Could you check a few things on this model? Use its own coordinates, in mm. Face numbers are marked on the shaded views. A direction names the side the tool comes from. Give positions to 0.01 mm unless a question says otherwise; leave off trailing zeros. Loops run counter-clockwise (first coordinate to the right, second up) from the corner with the lowest first, then second, coordinate; pieces in that order, holes last. Notation, with made-up numbers: (39, -7) - (78, -7) arc R31 cw to (78, 31) - close; hole circle Ø2 at (51, 52.5). An arc over 180 degrees is marked (long way). Write each question's results on one line, items separated by ' | '. Start each with the question number.
1) I'm going to push flat-ended pins straight in: pin 1 (1.1 mm diameter, centred on x = -1, z = 4.5, fed in from +Y); pin 2 (3 mm diameter, centred on x = 3, z = 1.5, fed in from +Y); pin 3 (0.8 mm diameter, centred on y = -1.5, z = 4.5, fed in from -X). Where does each tip first touch, or does it pass through?
2) If we mould it in two halves opening along Y, with no side actions, what happens to the marked faces 4, 5 and 6? For each: +Y half, -Y half, draft (parallel to the pull), parting line (faces both ways), or undercut.
3) I want a section at A-A, the plane z = 1.05. Write out the boundary of the cut face in (x, y).
4) On a 3-axis mill with a long thin cutter (end or side, diameter ignored), from which of +Z, -Z, +X, -X, +Y, -Y can I reach the whole of each face in a straight line? I mean the marked faces 1, 2 and 3. Say none if no direction works.
5) If I drill on probe 1 along Y at (x, z) = (0, 2.35); probe 2 along Y at (x, z) = (11, 2.9); probe 3 along X at (y, z) = (-1.5, 1.05), over which ranges is the centre line in solid material (lowest first)? Write a range as [from, to].
6) I want a section at B-B, the plane x = 0. Write out the boundary of the cut face in (y, z).
from build123d import *

# Parameters (mm, degrees)
SKETCH001_R     = 20
PAD_DEPTH       = 5
SKETCH_R        = 17.38
POCKET_DEPTH    = 3
CHAMFER_SIZE    = 0.5
SKETCH002_W     = 11.2
SKETCH002_H     = 11.2
POCKET001_DEPTH = 1


with BuildPart() as part:
    # Sketch001 → Pad (new body)
    with BuildSketch(Plane.XY):
        Circle(SKETCH001_R)
    extrude(amount=PAD_DEPTH)

    # Sketch → Pocket (cut)
    with BuildSketch(Plane.XY):
        Circle(SKETCH_R)
        with BuildLine():
            ThreePointArc((-6.55, 11.55), (-10.085534, 10.085534), (-11.55, 6.55))
            Line((-11.55, -6.55), (-11.55, 6.55))
            ThreePointArc((-11.55, -6.55), (-10.085534, -10.085534), (-6.55, -11.55))
            Line((6.55, -11.55), (-6.55, -11.55))
            ThreePointArc((6.55, -11.55), (10.085534, -10.085534), (11.55, -6.55))
            Line((11.55, 6.55), (11.55, -6.55))
            ThreePointArc((11.55, 6.55), (10.085534, 10.085534), (6.55, 11.55))
            Line((-6.55, 11.55), (6.55, 11.55))
        make_face(mode=Mode.SUBTRACT)
    extrude(amount=POCKET_DEPTH, mode=Mode.SUBTRACT)

    # Chamfer
    chamfer_edges = [part.edges().sort_by_distance(p)[0] for p in [
        (0, 11.55, 0),
        (10.085534, 10.085534, 0),
        (11.55, 0, 0),
        (10.085534, -10.085534, 0),
        (0, -11.55, 0),
        (-10.085534, -10.085534, 0),
        (-11.55, 0, 0),
        (-10.085534, 10.085534, 0),
        (-17.38, 0, 0),
        (-20, 0, 5),
    ]]
    chamfer(chamfer_edges, length=CHAMFER_SIZE)

    # Sketch002 (on DatumPlane) → Pocket001 (cut)
    with BuildSketch(Plane.XY.offset(5)):
        Rectangle(SKETCH002_W, SKETCH002_H)
    extrude(amount=-POCKET001_DEPTH, mode=Mode.SUBTRACT)


solid = part.part
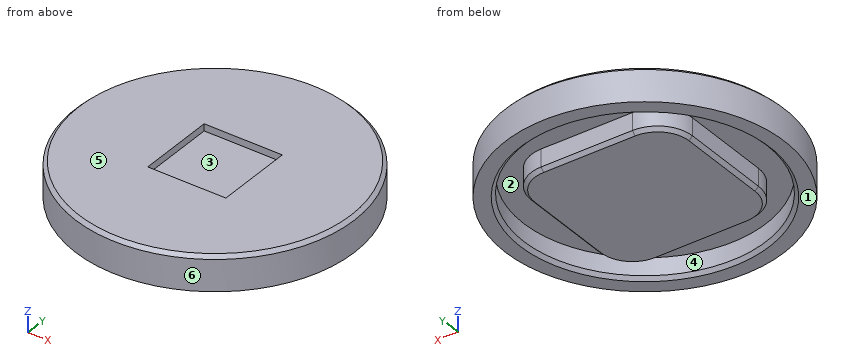
Answers:
1) pin 1: stops at y = 19.99 | pin 2: stops at y = 19.94 | pin 3: stops at x = -19.97
2) face 4: undercut | face 5: draft | face 6: parting line
3) outline: circle Ø40 at (0, 0); (-11.55, -6.55) arc R5 ccw to (-6.55, -11.55) - (6.55, -11.55) arc R5 ccw to (11.55, -6.55) - (11.55, 6.55) arc R5 ccw to (6.55, 11.55) - (-6.55, 11.55) arc R5 ccw to (-11.55, 6.55) - close; hole circle Ø34.76 at (0, 0)
4) face 1: -Z, +X, -X, +Y, -Y | face 2: -Z | face 3: +Z
5) probe 1: y = [-20, -17.38], [-11.55, 11.55], [17.38, 20] | probe 2: y = [-16.7, -13.46], [-8.83, 8.83], [13.46, 16.7] | probe 3: x = [-19.94, -17.32], [-11.55, 11.55], [17.32, 19.94]
6) outline: (-20, 0) - (-17.88, 0) - (-17.38, 0.5) - (-17.38, 3) - (-11.55, 3) - (-11.55, 0.5) - (-11.05, 0) - (11.05, 0) - (11.55, 0.5) - (11.55, 3) - (17.38, 3) - (17.38, 0.5) - (17.88, 0) - (20, 0) - (20, 4.5) - (19.5, 5) - (5.6, 5) - (5.6, 4) - (-5.6, 4) - (-5.6, 5) - (-19.5, 5) - (-20, 4.5) - close
